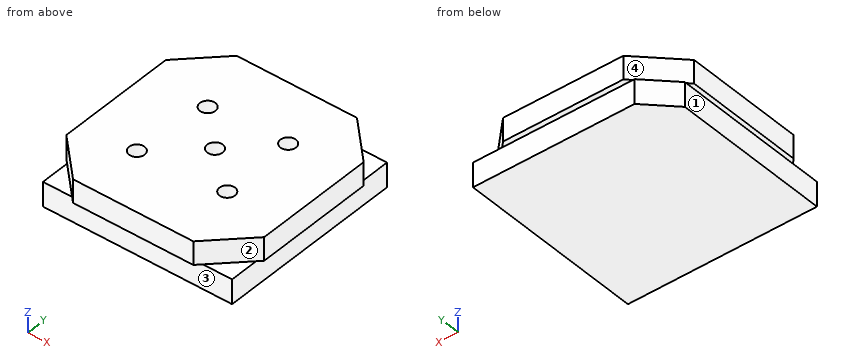
```python
from build123d import *

# Parameters (mm, degrees)
F0_W      = 64.756296
F0_H      = 64.756296
F1_DEPTH  = 7.62
F2_SIZE   = 12.7
F3_SIZE   = 12.7
F4_SIZE   = 12.7
F5_SIZE   = 12.7
F12_D     = 5.08
F13_D     = 5.08
F14_D     = 5.08
F15_D     = 5.08
F6_W      = 61.878238
F6_H      = 61.302628
F16_DEPTH = 8
F17_SIZE  = 9


with BuildPart() as f1:
    # F0 (on Top) → F1 (new body)
    with BuildSketch(Plane.XY):
        Rectangle(F0_W, F0_H)
    extrude(amount=F1_DEPTH)

    # F2
    f2_edges = [f1.edges().sort_by_distance(p)[0] for p in [
        (32.378148, -32.378148, 3.81),
    ]]
    chamfer(f2_edges, length=F2_SIZE)

    # F3
    f3_edges = [f1.edges().sort_by_distance(p)[0] for p in [
        (-32.378148, 32.378148, 3.81),
    ]]
    chamfer(f3_edges, length=F3_SIZE)

    # F4
    f4_edges = [f1.edges().sort_by_distance(p)[0] for p in [
        (-32.378148, -32.378148, 3.81),
    ]]
    chamfer(f4_edges, length=F4_SIZE)

    # F5
    f5_edges = [f1.edges().sort_by_distance(p)[0] for p in [
        (32.378148, 32.378148, 3.81),
    ]]
    chamfer(f5_edges, length=F5_SIZE)

    # F12 (through all)
    with Locations(Plane(origin=(0, 0, 0), x_dir=(1, 0, 0), z_dir=(0, 0, -1))):
        with Locations((13.451747, 11.412409)):
            Hole(F12_D / 2)

    # F13 (through all)
    with Locations(Plane(origin=(0, 0, 0), x_dir=(1, 0, 0), z_dir=(0, 0, -1))):
        with Locations((12.937722, -13.321196)):
            Hole(F13_D / 2)

    # F14 (through all)
    with Locations(Plane(origin=(0, 0, 0), x_dir=(1, 0, 0), z_dir=(0, 0, -1))):
        with Locations((0, 0)):
            Hole(F14_D / 2)

    # F15 (through all)
    with Locations(Plane(origin=(0, 0, 0), x_dir=(1, 0, 0), z_dir=(0, 0, -1))):
        with Locations((-12.155064, -11.785694), (-14.640464, 13.230935)):
            Hole(F15_D / 2)

    # F6 (on Top) → F16 (join)
    with BuildSketch(Plane.XY):
        Rectangle(F6_W, F6_H)
    extrude(amount=-F16_DEPTH)

    # F17
    f17_edges = [f1.edges().sort_by_distance(p)[0] for p in [
        (-30.939119, 30.651314, -4),
    ]]
    chamfer(f17_edges, length=F17_SIZE)


solid = f1.part
```
Here's how the part is built. I have some questions about the finished solid (model axes, mm). Face numbers are marked on the shaded views. A direction names the side the tool comes from. Coordinates: 2 decimals unless noted, no trailing zeros. Order: outer loops, then holes, each group sorted by start corner. A loop starts at its lowest first (then second) coordinate and runs counter-clockwise, first axis right, second up.
Item 1: If we section it at C-C, the plane z = 4.75: List the corners of the cut face in (x, y) for me, then the cut area to 3 significant figures.
Response values:
outline: (-32.38, -19.68) - (-19.68, -32.38) - (19.68, -32.38) - (32.38, -19.68) - (32.38, 19.68) - (19.68, 32.38) - (-19.68, 32.38) - (-32.38, 19.68) - close; hole circle Ø5.08 at (-14.64, -13.23); hole circle Ø5.08 at (-12.16, 11.79); hole circle Ø5.08 at (0, 0); hole circle Ø5.08 at (12.94, 13.32); hole circle Ø5.08 at (13.45, -11.41)
area: 3,770 mm2
Item 2: Which directions (+Z, -Z, +X, -X, +Y, -Y) give clear straight access to the entire face, cutting with the end or side of a thin tool? Please do the marked faces 1, 2, 3 and 4.
Response values:
face 1: -Z, -X, +Y, -Y
face 2: +Z, +X, -Y
face 3: -Z, +X, -X, -Y
face 4: +Z, -X, +Y
Item 3: I need wall thicknesses on probe 1 along Y at (x, z) = (0, 4); probe 2 along X at (y, z) = (12, 2.75); probe 3 along Y at (x, z) = (-12, 6.75). Which ranges of each line are inside material? Lowest first, please.
Response values:
probe 1: y = -32.38 to -2.54, 2.54 to 32.38
probe 2: x = -32.38 to -14.69, -9.62 to 10.77, 15.11 to 32.38
probe 3: y = -32.38 to 9.25, 14.32 to 32.38
Item 4: If we section it at D-D, the plane z = -5: List the corners of the cut face in (x, y) for me.
Response values:
outline: (-30.94, -30.65) - (30.94, -30.65) - (30.94, 30.65) - (-21.94, 30.65) - (-30.94, 21.65) - close
Item 5: I'm going to push flat-ended pins straight in: pin 1 Ø5 at (y, z) = (-22.5, -4.5) entering from -X; pin 2 Ø6.5 at (y, z) = (0.5, -4) entering from +X; pin 3 Ø1 at (x, z) = (2, -5) entering from +Y. Where does each tip first touch, or does it pass through?
Response values:
pin 1: stops at x = -30.94
pin 2: stops at x = 30.94
pin 3: stops at y = 30.65
Item 6: If we section it at B-B, the plane x = 0: List the corners of the cut face in (y, z) for me.
Response values:
outline: (-32.38, 0) - (-30.65, 0) - (-30.65, -8) - (30.65, -8) - (30.65, 0) - (32.38, 0) - (32.38, 7.62) - (2.54, 7.62) - (2.54, 0) - (-2.54, 0) - (-2.54, 7.62) - (-32.38, 7.62) - close
Item 7: If we section it at A-A, the plane y = -4: List the corners of the cut face in (x, z) for me, then the cut area to 3 significant figures.
Response values:
outline: (-32.38, 0) - (-30.94, 0) - (-30.94, -8) - (30.94, -8) - (30.94, 0) - (32.38, 0) - (32.38, 7.62) - (-32.38, 7.62) - close
area: 988 mm2
